Input: part model. Units: mm. Frame: model coordinates. A direction names the side the tool comes from. Round coordinates to 2 decimals unless told otherwise and drop trailing zeros. Order: outer loops, then holes, each group sorted by start corner. A loop starts at its lowest first (then second) coordinate and runs counter-clockwise, first axis right, second up. Notation, with made-up numbers: (56.25, 39.25) -> (102.25, 39.25) arc R30 ccw to (102.25, 69.25) -> close; hole circle Ø4 at (45, 34.25). An arc over 180 degrees is marked (long way). Use a Markdown table: item, result.
from build123d import *

# Parameters (mm, degrees)
F1_DEPTH = 35
F2_R     = 2.5
F3_DEPTH = 35.001
F4_DEPTH = 35
F6_DEPTH = 30


with BuildPart() as f1:
    # F0 (on Front) → F1 (new body, symmetric)
    with BuildSketch(Plane.XZ):
        with BuildLine():
            ThreePointArc((-25, 0), (0, 25), (25, 0))
            Line((25, 0), (25, 35))
            Line((25, 35), (-25, 35))
            Line((-25, 35), (-25, 0))
        make_face()
        with BuildLine():
            Line((23, 0), (25, 0))
            ThreePointArc((25, 0), (0, 25), (-25, 0))
            Line((-25, 0), (-23, 0))
            ThreePointArc((-23, 0), (0, 23), (23, 0))
        make_face()
    extrude(amount=F1_DEPTH, both=True)

    # F2 (on face) → F3 (cut, through all)
    with BuildSketch(Plane.XY.offset(35)):
        with Locations((20, 20)):
            Circle(F2_R)
        with Locations((-20, 20)):
            Circle(F2_R)
        with Locations((-20, -20)):
            Circle(F2_R)
        with Locations((20, -20)):
            Circle(F2_R)
    extrude(amount=-F3_DEPTH, mode=Mode.SUBTRACT)

    # F0 (on Front) → F4 (join, symmetric)
    with BuildSketch(Plane.XZ):
        with BuildLine():
            ThreePointArc((-25, 0), (0, -25), (25, 0))
            Line((25, 0), (23, 0))
            ThreePointArc((23, 0), (0, -23), (-23, 0))
            Line((-23, 0), (-25, 0))
        make_face()
    extrude(amount=F4_DEPTH, both=True)

    # F5 (on Top) → F6 (cut)
    with BuildSketch(Plane.XY):
        Polygon((-17.1132486541, -20), (-18.556624327, -17.5), (-21.443375673, -17.5), (-22.8867513459, -20), (-21.443375673, -22.5), (-18.556624327, -22.5), align=None)
        Polygon((21.443375673, -17.5), (18.556624327, -17.5), (17.1132486541, -20), (18.556624327, -22.5), (21.443375673, -22.5), (22.8867513459, -20), align=None)
        Polygon((-21.443375673, 17.5), (-18.556624327, 17.5), (-17.1132486541, 20), (-18.556624327, 22.5), (-21.443375673, 22.5), (-22.8867513459, 20), align=None)
        Polygon((17.1132486541, 20), (18.556624327, 17.5), (21.443375673, 17.5), (22.8867513459, 20), (21.443375673, 22.5), (18.556624327, 22.5), align=None)
    extrude(amount=F6_DEPTH, mode=Mode.SUBTRACT)


solid = f1.part
1) Cut plane C-C on y = -16.5. Return loops of the section in (x, z), and give its area (3 significant figures).
Results found:
| item | result |
|---|---|
| outline | (-25, 0) arc R25 ccw to (25, 0) -> (25, 35) -> (-25, 35) -> close; hole circle Ø46 at (0, 0) |
| area | 1,070 mm² |
2) Cut plane D-D on z = -9.5. Return loops of the section in (x, y).
Results found:
| item | result |
|---|---|
| outline | (-23.12, -35) -> (-20.95, -35) -> (-20.95, 35) -> (-23.12, 35) -> close; (20.95, -35) -> (23.12, -35) -> (23.12, 35) -> (20.95, 35) -> close |
3) Cut plane B-B on z = 27. Return loops of the section in (x, y).
Results found:
| item | result |
|---|---|
| outline | (-25, -35) -> (25, -35) -> (25, 35) -> (-25, 35) -> close; hole (-22.89, -20) -> (-21.44, -22.5) -> (-18.56, -22.5) -> (-17.11, -20) -> (-18.56, -17.5) -> (-21.44, -17.5) -> close; hole (-22.89, 20) -> (-21.44, 17.5) -> (-18.56, 17.5) -> (-17.11, 20) -> (-18.56, 22.5) -> (-21.44, 22.5) -> close; hole (17.11, -20) -> (18.56, -22.5) -> (21.44, -22.5) -> (22.89, -20) -> (21.44, -17.5) -> (18.56, -17.5) -> close; hole (17.11, 20) -> (18.56, 17.5) -> (21.44, 17.5) -> (22.89, 20) -> (21.44, 22.5) -> (18.56, 22.5) -> close |
4) Cut plane A-A on x = 0. Return loops of the section in (y, z).
Results found:
| item | result |
|---|---|
| outline | (-35, -25) -> (35, -25) -> (35, -23) -> (-35, -23) -> close; (-35, 23) -> (35, 23) -> (35, 35) -> (-35, 35) -> close |
5) Set-up query: faces 1 (the cylindrical face through (-2.994, -0.49, -22.804)), 2 (the cylindrical face through (17.5, -19.9, 32.5)), 3 (the flat face through (22.155, 18.732, 19.026)). Return all of +Z, -Z, +X, -X, +Y, -Y with unobstructed straight access to the full face (end or side cutting, diameter ignored); none if empty.
Results found:
| item | result |
|---|---|
| face 1 | +Y, -Y |
| face 2 | +Z |
| face 3 | none |
6) Pin query (flat end, axial travel): pin 1 Ø1.4 at (x, y) = (19, -18) entering from -Z; pin 2 Ø10 at (y, z) = (-14.5, -7) entering from -X; pin 3 Ø2 at (y, z) = (4.5, -17.5) entering from -X; pin 4 Ø12 at (x, z) = (-2.5, -16) entering from +Y. Return the tip coordinate at first contact, or that it passes through.
Results found:
| item | result |
|---|---|
| pin 1 | stops at z = -17.03 |
| pin 2 | stops at x = -24.92 |
| pin 3 | stops at x = -18.78 |
| pin 4 | passes through |
7) Line query: L1, parallel to X at y = -20, z = 31; L2, parallel to Y at x = 20, z = 32; L3, parallel to X at y = 21, z = 30. Output: solid intervals per line, ascending. Write a range as [from, to].
Results found:
| item | result |
|---|---|
| L1 | x = [-25, -22.5], [-17.5, 17.5], [22.5, 25] |
| L2 | y = [-35, -22.5], [-17.5, 17.5], [22.5, 35] |
| L3 | x = [-25, -22.31], [-17.69, 17.69], [22.31, 25] |
8) Pull-direction query (Z, two-part tool) for faces 4 (the flat face through (0, 0, 35)), 5 (the flat face through (-22.175, 18.768, 19.026)), 6 (the flat face through (5, 35, 23)); classes: +Z half, -Z half, draft (parallel to the pull), parting line (faces both ways), or undercut.
Results found:
| item | result |
|---|---|
| face 4 | +Z half |
| face 5 | undercut |
| face 6 | draft |
